Here's how the part is built. I have some questions about the finished solid (model axes, mm). A direction names the side the tool comes from. Give positions to 0.01 mm unless a question says otherwise; leave off trailing zeros. Loops run counter-clockwise (first coordinate to the right, second up) from the corner with the lowest first, then second, coordinate; pieces in that order, holes last. Notation, with made-up numbers: (78.25, 48.25) -> (88.25, 48.25) arc R21 cw to (88.25, 77.25) -> close; hole circle Ø8 at (-23, 62.25). An arc over 180 degrees is marked (long way). Answer in a Markdown table with one row per item. Add a question column.
Item 1: We'd pull the mould along Y, two halves only. Please class faces 1 (the face through (2, 68.611, 50)), 2 (the face through (2, 74.961, 50)), 3 (the face through (27.464, 17, 50)), 4 (the face through (28, 22, 101.6)): released by +Y, released by -Y, zero draft, split by the parting line, or undercut.
Item 2: If I drill on line 1 (Y direction, x = 16, z = 77.5); line 2 (X direction, y = 39.5, z = 59); line 3 (Y direction, x = 28.5, z = 29), over which ranges is the centre line in solid material (lowest first)?
Item 3: If we section it at A-A (x = -4.5): Write out the boundary of the cut face in (y, z).
Item 4: If we section it at C-C (z = 64): Write out the boundary of the cut face in (x, y).
Item 5: If we section it at B-B (y = 43.5): Write out the boundary of the cut face in (x, z), then the cut area to 3 significant figures.
Item 6: If we section it at D-D (y = 61): Write out the boundary of the cut face in (x, z), then the cut area to 3 significant figures.
Item 7: Which directions (+Z, -Z, +X, -X, +Y, -Y) give clear straight access to the entire face, cutting with the end or side of a thin tool? Please do faces 5 (the face through (2, -39.822, 50)), 6 (the face through (31, 2.119, 21)), 7 (the face through (-23.336, 17, 50)).
```python
from build123d import *

# Parameters (mm, degrees)
F0_W     = 63.5
F0_H     = 114.7826
F0_W_2   = 50.8
F0_H_2   = 102.0826
F1_DEPTH = 101.6
F2_W     = 50.8
F2_H     = 25.4
F3_DEPTH = 25.4


with BuildPart() as f1:
    # F0 (on Top) → F1 (new body)
    with BuildSketch(Plane.XY):
        with Locations((2.064243, 17.569714)):
            Rectangle(F0_W, F0_H)
        with Locations((2.064243, 17.569714)):
            Rectangle(F0_W_2, F0_H_2, mode=Mode.SUBTRACT)
    extrude(amount=F1_DEPTH)

    # F2 (on face) → F3 (cut)
    with BuildSketch(Plane.YZ.offset(33.814243)):
        with Locations((27.519288, 21.59)):
            Rectangle(F2_W, F2_H)
    extrude(amount=-F3_DEPTH, mode=Mode.SUBTRACT)


solid = f1.part
```
Recorded:
| question | item | result |
|---|---|---|
| 1 | face 1 | undercut |
| 1 | face 2 | released by +Y |
| 1 | face 3 | undercut |
| 1 | face 4 | zero draft |
| 2 | line 1 | y = -39.82 to -33.47, 68.61 to 74.96 |
| 2 | line 2 | x = -29.69 to -23.34, 27.46 to 33.81 |
| 2 | line 3 | y = -39.82 to 2.12, 52.92 to 74.96 |
| 3 | outline | (-39.82, 0) -> (-33.47, 0) -> (-33.47, 101.6) -> (-39.82, 101.6) -> close; (68.61, 0) -> (74.96, 0) -> (74.96, 101.6) -> (68.61, 101.6) -> close |
| 4 | outline | (-29.69, -39.82) -> (33.81, -39.82) -> (33.81, 74.96) -> (-29.69, 74.96) -> close; hole (-23.34, -33.47) -> (27.46, -33.47) -> (27.46, 68.61) -> (-23.34, 68.61) -> close |
| 5 | outline | (-29.69, 0) -> (-23.34, 0) -> (-23.34, 101.6) -> (-29.69, 101.6) -> close; (27.46, 0) -> (33.81, 0) -> (33.81, 8.89) -> (27.46, 8.89) -> close; (27.46, 34.29) -> (33.81, 34.29) -> (33.81, 101.6) -> (27.46, 101.6) -> close |
| 5 | area | 1,130 mm^2 |
| 6 | outline | (-29.69, 0) -> (-23.34, 0) -> (-23.34, 101.6) -> (-29.69, 101.6) -> close; (27.46, 0) -> (33.81, 0) -> (33.81, 101.6) -> (27.46, 101.6) -> close |
| 6 | area | 1,290 mm^2 |
| 7 | face 5 | +Z, -Z, +X, -X, -Y |
| 7 | face 6 | +X |
| 7 | face 7 | +Z, -Z |
